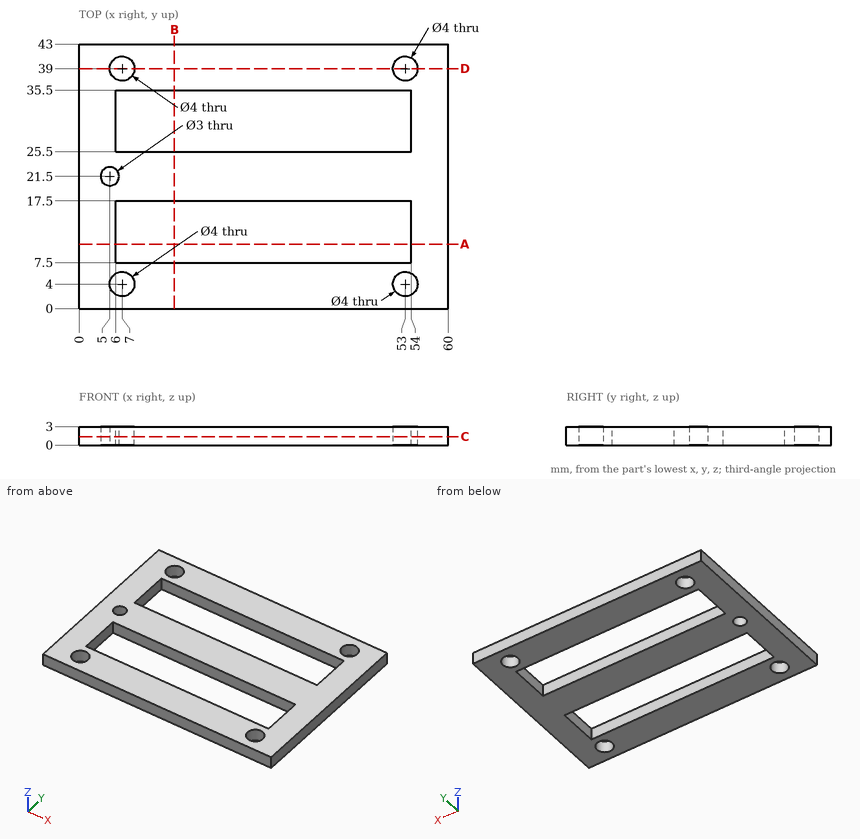
Input: dimensioned drawing with shaded views. Units: mm. Origin: part minimum x, y, z. Give positions to 0.01 mm unless a question says otherwise; leave off trailing zeros. Write each loop counter-clockwise with the first axis right and the second up, starting at its lowest first coordinate (ties: lowest second). Pieces come first, ordered by that corner, then holes.
Q1. Material intervals for probe 1 along Y at (x, z) = (14.5, 2); probe 2 along Y at (x, z) = (7, 0.9); probe 3 along X at (y, z) = (4, 1.1), sorted ascending.
Q2. First-contact query: P1, Ø1.5, axis at x = 27.5, y = 17, coming from the +Z side; P2, Ø2.5, axis at x = 53, y = 39, coming from the +Z side. Flat tips, straight axial feed; report the tip coordinate or a pass-through.
Q3. Section B-B, the plane x = 15.5. Output: boundary loops of the cut face in (y, z).
Q4. Section A-A, the plane y = 10.5. Output: boundary loops of the cut face in (x, z).
Q5. Section C-C, the plane z = 1.4. Output: boundary loops of the cut face in (x, y), plus the area to 3 significant figures.
Q6. Section D-D, the plane y = 39. Output: boundary loops of the cut face in (x, z).
Filled in:
1. probe 1: y = 0 to 7.5, 17.5 to 25.5, 35.5 to 43
1. probe 2: y = 0 to 2, 6 to 7.5, 17.5 to 25.5, 35.5 to 37, 41 to 43
1. probe 3: x = 0 to 5, 9 to 51, 55 to 60
2. P1: stops at z = 3
2. P2: passes through
3. outline: (0, 0) - (7.5, 0) - (7.5, 3) - (0, 3) - close; (17.5, 0) - (25.5, 0) - (25.5, 3) - (17.5, 3) - close; (35.5, 0) - (43, 0) - (43, 3) - (35.5, 3) - close
4. outline: (0, 0) - (6, 0) - (6, 3) - (0, 3) - close; (54, 0) - (60, 0) - (60, 3) - (54, 3) - close
5. outline: (0, 0) - (60, 0) - (60, 43) - (0, 43) - close; hole circle Ø3 at (5, 21.5); hole circle Ø4 at (7, 4); hole circle Ø4 at (7, 39); hole (6, 7.5) - (54, 7.5) - (54, 17.5) - (6, 17.5) - close; hole (6, 25.5) - (54, 25.5) - (54, 35.5) - (6, 35.5) - close; hole circle Ø4 at (53, 4); hole circle Ø4 at (53, 39)
5. area: 1,560 mm2
6. outline: (0, 0) - (5, 0) - (5, 3) - (0, 3) - close; (9, 0) - (51, 0) - (51, 3) - (9, 3) - close; (55, 0) - (60, 0) - (60, 3) - (55, 3) - close
